Design review of the part shown in the three views and the two pictorial views. Dimensions are in mm from the part's minimum x, y and z. Give positions to 0.01 mm unless a question says otherwise; leave off trailing zeros. Write each loop counter-clockwise with the first axis right and the second up, starting at its lowest first coordinate (ties: lowest second). Pieces come first, ordered by that corner, then holes. Notation, with made-up numbers: M 36,29 L 53,29 A22 ccw 53,62 Z; hole C -35.5,70.25 d6. An arc over 180 degrees is marked long. Write item = value, one per line.
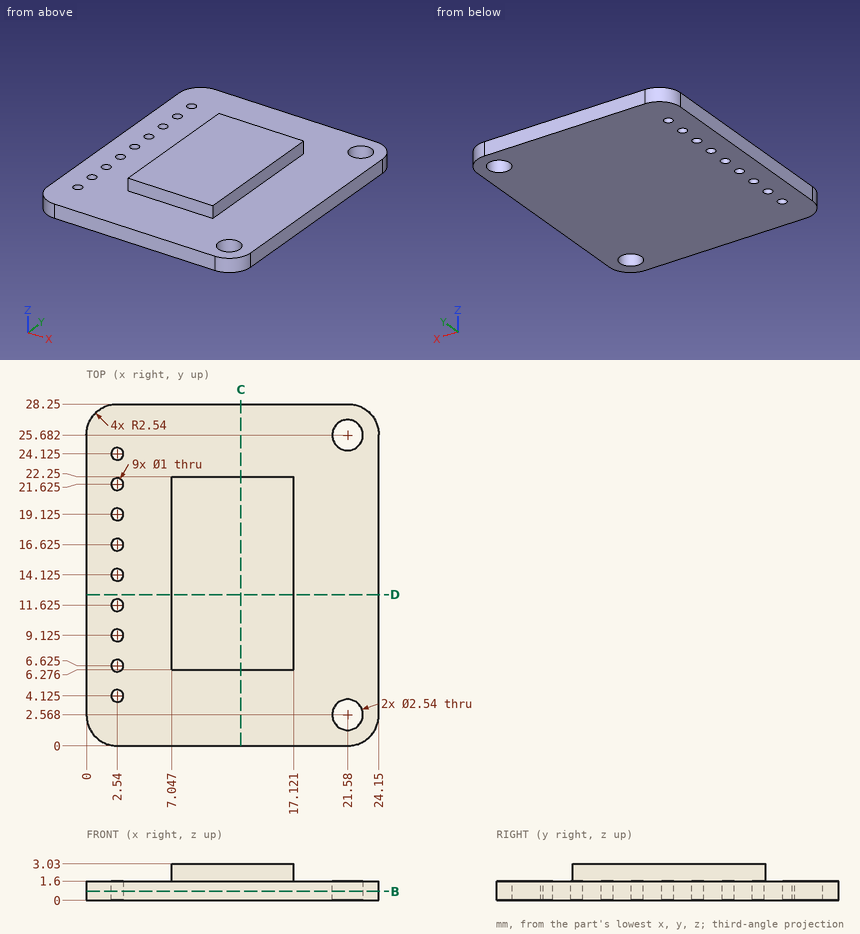
1. For line 1 along X through (y, z) = (18, 2.5); line 2 along Z through (x, y) = (16.75, 23.5); line 3 along Y through (x, z) = (9.25, 2.05), list the stretches that pass through material, from the lowest coordinate up. Write a range as from..to.
Responses:
line_1 = 7.05..17.12
line_2 = 0..1.6
line_3 = 6.28..22.25
2. We need section D-D, the plane y = 12.5. Write out the cut boundary in (x, z).
Responses:
outline = M 0,0 L 24.15,0 L 24.15,1.6 L 17.12,1.6 L 17.12,3.03 L 7.05,3.03 L 7.05,1.6 L 0,1.6 Z
3. Insertion check: P1, Ø1.1, axis at x = 11.5, z = 2.5, coming from the -Y side; P2, Ø5, axis at x = 21, y = 10.5, coming from the +Z side; P3, Ø0.7, axis at x = 12.5, z = 2.5, coming from the +Y side. Each pin has a flat end and moves straight along its axis. Give the tip position at first contact, or say it passes through.
Responses:
P1 = 6.28
P2 = 1.6
P3 = 22.25
4. We need section B-B, the plane z = 0.75. Count the separate pieces of the cut face and the enclosed holes in it.
Responses:
separate_pieces = 1
enclosed_holes = 11
5. We need section C-C, the plane x = 12.75. Write out the cut boundary in (y, z).
Responses:
outline = M 0,0 L 28.25,0 L 28.25,1.6 L 22.25,1.6 L 22.25,3.03 L 6.28,3.03 L 6.28,1.6 L 0,1.6 Z
